The model under review builds one solid part; all positions refer to its coordinate system, in mm. Face numbers are marked on the shaded views. A direction names the side the tool comes from. Coordinates: 2 decimals unless noted, no trailing zeros. Order: outer loops, then holes, each group sorted by start corner. A loop starts at its lowest first (then second) coordinate and runs counter-clockwise, first axis right, second up. Notation, with made-up numbers: (51.5, 5) -> (90.5, 5) arc R25 cw to (90.5, 19) -> close; hole circle Ø7 at (88, 71.25). An arc over 180 degrees is marked (long way). Use one line per item in the form item = value. Start each with the question number.
(1) Take a section at C-C (x = 5). State the section outline as (y, z) points.
(2) Wall thickness on line 1 along X through (y, z) = (1.7, 0) (3 decimals); line 2 along Z through (x, y) = (-5.5, 0.05); line 3 along Y through (x, z) = (-3.5, -5.5): over which ranges is each line inside the solid? List them lowest first.
(3) Take a section at D-D (y = 4.35). State the section outline as (x, z) points (3 decimals).
(4) Insertion check: pin 1 Ø4 at (x, z) = (-2, 1.5) entering from +Y; pin 2 Ø2 at (x, y) = (0.5, 3.5) entering from -Z. Each pin has a flat end and moves straight along its axis. Give the tip position at first contact, or say it passes through.
(5) Take a section at A-A (z = 0). State the section outline as (x, y) points (3 decimals), then the cut area to 3 significant figures.
(6) Take a section at B-B (x = 0). State the section outline as (y, z) points (3 decimals).
(7) Mouldability with a two-part tool opening along X and no side actions: class the marked faces 3, 4 and 5 as +X half, -X half, draft (parallel to the pull), parting line (faces both ways), or undercut.
(8) For the marked faces 1 and 2, list the 3-axis set-ups (+Z, -Z, +X, -X, +Y, -Y) from which the entire face can be reached by the end or side of a thin tool; tool diameter is ignored.
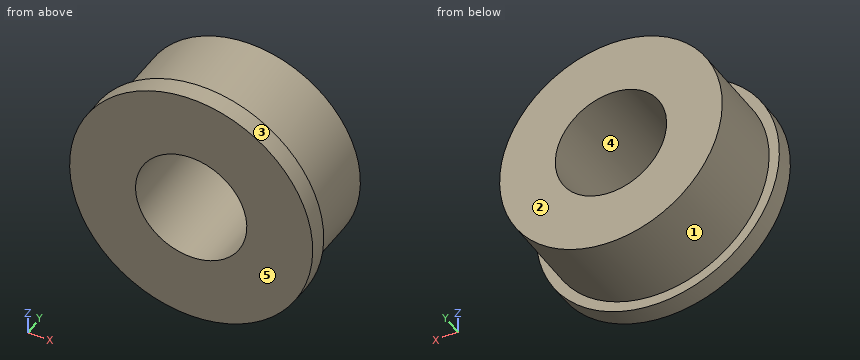
```python
from build123d import *

# Parameters (mm, degrees)
SKETCH1_R           = 6.35
BOSS_EXTRUDE1_DEPTH = 4.7498
SKETCH2_R           = 6.9342
BOSS_EXTRUDE2_DEPTH = 1.1176
CUT_EXTRUDE1_REACH  = 13.428
SKETCH3_R           = 3.175


with BuildPart() as part:
    # Sketch1 → Boss-Extrude1 (new body)
    with BuildSketch(Plane(origin=(0, 0, 0), x_dir=(1, 0, 0), z_dir=(0, 1, 0))):
        with Locations(Location((0, 0, 0), (0, 0, 270))):
            Circle(SKETCH1_R)
    extrude(amount=BOSS_EXTRUDE1_DEPTH)

    # Sketch2 → Boss-Extrude2 (add)
    with BuildSketch(Plane.XZ):
        with Locations(Location((0, 0, 0), (0, 0, 270))):
            Circle(SKETCH2_R)
    extrude(amount=BOSS_EXTRUDE2_DEPTH)

    # Sketch3 → Cut-Extrude1 (cut, up to next)
    with BuildSketch(Plane(origin=(0, 4.7498, 0), x_dir=(1, 0, 0), z_dir=(0, 1, 0)), mode=Mode.PRIVATE) as cut_extrude1_sk1:
        with Locations(Location((0, 0, 0), (0, 0, 270))):
            Circle(SKETCH3_R)
    cut_extrude1_tool1 = extrude(cut_extrude1_sk1.sketch, amount=-CUT_EXTRUDE1_REACH, mode=Mode.PRIVATE) & part.part
    add(cut_extrude1_tool1.solids().sort_by_distance((0, 4.7498, 0))[0], mode=Mode.SUBTRACT)


solid = part.part
```
Findings:
q1.outline = (-1.12, -4.8) -> (0, -4.8) -> (0, -3.91) -> (4.75, -3.91) -> (4.75, 3.91) -> (0, 3.91) -> (0, 4.8) -> (-1.12, 4.8) -> close
q2.line_1 = -6.35 to -3.175, 3.175 to 6.35
q2.line_2 = -3.17 to 3.17
q2.line_3 = -1.12 to 0
q3.outline = circle Ø12.7 at (0, 0); hole circle Ø6.35 at (0, 0)
q4.pin_1 = 4.75
q4.pin_2 = -6.35
q5.outline = (-6.934, -1.118) -> (-3.175, -1.118) -> (-3.175, 4.75) -> (-6.35, 4.75) -> (-6.35, 0) -> (-6.934, 0) -> close; (3.175, -1.118) -> (6.934, -1.118) -> (6.934, 0) -> (6.35, 0) -> (6.35, 4.75) -> (3.175, 4.75) -> close
q5.area = 38.6 mm²
q6.outline = (-1.118, -6.934) -> (0, -6.934) -> (0, -6.35) -> (4.75, -6.35) -> (4.75, -3.175) -> (-1.118, -3.175) -> close; (-1.118, 3.175) -> (4.75, 3.175) -> (4.75, 6.35) -> (0, 6.35) -> (0, 6.934) -> (-1.118, 6.934) -> close
q7.face_3 = parting line
q7.face_4 = undercut
q7.face_5 = draft
q8.face_1 = +Y
q8.face_2 = +Z, -Z, +X, -X, +Y
